Source: CAD feature listing. Evaluate the final solid. Frame: model axes, mm. Coordinates: 2 decimals unless noted, no trailing zeros. Order: outer loops, then holes, each group sorted by start corner. A loop starts at its lowest first (then second) coordinate and runs counter-clockwise, first axis right, second up. Notation, with made-up numbers: (32, -8.75) -> (68, -8.75) arc R25 ccw to (68, 8.25) -> close; hole circle Ø10 at (-5.5, 0). An arc over 180 degrees is marked (long way). Write each question's results on one line, items separated by ' | '. Start each with the question number.
Solid Edge part; units mm, degrees
sketch "Sketch1" plane through (0, 0, 0) normal (0, 0, 1) x (1, 0, 0)
  line L0 (57.1488, -10.4) -> (57.1487, 0)
  arc A0 (56.1487, -11.4) -> (57.1487, -10.4) centre (56.1487, -10.4) ccw
  line L1 (-56.1487, -11.4) -> (56.1487, -11.4)
  arc A1 (-57.1487, -10.4) -> (-56.1487, -11.4) centre (-56.1487, -10.4) ccw
  line L2 (-57.1487, 0) -> (-57.1487, -10.4)
sketch "Sketch2" plane through (0, 0, 0) normal (0, -1, 0) x (1, 0, 0)
  circle A0 centre (57.1487, 0) radius 0.8
sweep "Geführte_Ausprägung_1" add profiles "Sketch2" path "Sketch1"
(1) First-contact query: P1, Ø2, axis at x = -8.5, y = -8, coming from the -Z side. Flat tip, straight axial feed; report the tip coordinate or a pass-through.
(2) Line query: L1, parallel to X at y = -8.75, z = -0.15; L2, parallel to Y at x = -36.5, z = 0.05; L3, parallel to X at y = -2.75, z = -0.45. Output: solid intervals per line, ascending.
(3) Section A-A on y = -3.5. Return the cut outline in (x, z), then the cut area to 3 significant figures.
(4) Section C-C on x = 32. Return the cut outline in (y, z), then the cut area to 3 significant figures.
(5) Section B-B on z = 0. Return the cut outline in (x, y), then the cut area to 3 significant figures.
Results list:
1) P1: passes through
2) L1: x = -57.93 to -56.36, 56.36 to 57.93 | L2: y = -12.2 to -10.6 | L3: x = -57.81 to -56.49, 56.49 to 57.81
3) outline: circle Ø1.6 at (-57.15, 0); circle Ø1.6 at (57.15, 0) | area: 4.02 mm²
4) outline: circle Ø1.6 at (-11.4, 0) | area: 2.01 mm²
5) outline: (-57.95, -10.4) arc R1.8 ccw to (-56.15, -12.2) -> (56.15, -12.2) arc R1.8 ccw to (57.95, -10.4) -> (57.95, 0) -> (56.35, 0) -> (56.35, -10.4) arc R0.2 cw to (56.15, -10.6) -> (-56.15, -10.6) arc R0.2 cw to (-56.35, -10.4) -> (-56.35, 0) -> (-57.95, 0) -> close | area: 218 mm²
